```python
from build123d import *

# Parameters (mm, degrees)
CORTE_EXTRUS_O1_REACH = 512
ESBO_O2_R             = 4.5


with BuildPart() as part:
    # Esboço1 → Revolução1 (revolve)
    with BuildSketch(Plane.XY):
        Polygon((0, 510), (173, 510), (173, 500), (136.525, 500), (136.525, 0), (125.955, 0), (125.955, 10), (131.955, 10), (131.955, 500), (0, 500), align=None)
    revolve(axis=Axis((0, 0, 0), (0, 1, 0)))

    # Esboço2 → Corte-extrusão1 (cut, up to next)
    with BuildSketch(Plane(origin=(0, 510, 0), x_dir=(1, 0, 0), z_dir=(0, 1, 0)), mode=Mode.PRIVATE) as corte_extrus_o1_sk1:
        with Locations((0, 30)):
            Circle(ESBO_O2_R)
    corte_extrus_o1_tool1 = extrude(corte_extrus_o1_sk1.sketch, amount=-CORTE_EXTRUS_O1_REACH, mode=Mode.PRIVATE) & part.part
    add(corte_extrus_o1_tool1.solids().sort_by_distance((0, 510, -30))[0], mode=Mode.SUBTRACT)
    # Esboço2 → Corte-extrusão1 (cut, up to next)
    with BuildSketch(Plane(origin=(0, 510, 0), x_dir=(1, 0, 0), z_dir=(0, 1, 0)), mode=Mode.PRIVATE) as corte_extrus_o1_sk2:
        with Locations((30, 0)):
            Circle(ESBO_O2_R)
    corte_extrus_o1_tool2 = extrude(corte_extrus_o1_sk2.sketch, amount=-CORTE_EXTRUS_O1_REACH, mode=Mode.PRIVATE) & part.part
    add(corte_extrus_o1_tool2.solids().sort_by_distance((30, 510, 0))[0], mode=Mode.SUBTRACT)
    # Esboço2 → Corte-extrusão1 (cut, up to next)
    with BuildSketch(Plane(origin=(0, 510, 0), x_dir=(1, 0, 0), z_dir=(0, 1, 0)), mode=Mode.PRIVATE) as corte_extrus_o1_sk3:
        with Locations((0, -30)):
            Circle(ESBO_O2_R)
    corte_extrus_o1_tool3 = extrude(corte_extrus_o1_sk3.sketch, amount=-CORTE_EXTRUS_O1_REACH, mode=Mode.PRIVATE) & part.part
    add(corte_extrus_o1_tool3.solids().sort_by_distance((0, 510, 30))[0], mode=Mode.SUBTRACT)
    # Esboço2 → Corte-extrusão1 (cut, up to next)
    with BuildSketch(Plane(origin=(0, 510, 0), x_dir=(1, 0, 0), z_dir=(0, 1, 0)), mode=Mode.PRIVATE) as corte_extrus_o1_sk4:
        with Locations((-30, 0)):
            Circle(ESBO_O2_R)
    corte_extrus_o1_tool4 = extrude(corte_extrus_o1_sk4.sketch, amount=-CORTE_EXTRUS_O1_REACH, mode=Mode.PRIVATE) & part.part
    add(corte_extrus_o1_tool4.solids().sort_by_distance((-30, 510, 0))[0], mode=Mode.SUBTRACT)


solid = part.part
```
Geometry check sheet. Reference: the model listing, model coordinates, mm. A direction names the side the tool comes from. Coordinates: 2 decimals unless noted, no trailing zeros. Order: outer loops, then holes, each group sorted by start corner. A loop starts at its lowest first (then second) coordinate and runs counter-clockwise, first axis right, second up.
Item 1: Scan lines: line 1 along Z through (x, y) = (0, 505); line 2 along X through (y, z) = (6.5, 0) (3 decimals). Record each from-to range of solid material in increasing order.
Item 2: Section check D-D (x = 152). Enter the section's corners in (y, z), plus the area to 3 significant figures.
Item 3: Mould release check, pull along X, two halves, no side actions. Record for faces 1 (the cylindrical face through (125.86, 258.43, -39.64)), 2 (the flat face through (127, 500, -52)), 3 (the cylindrical face through (-137.287, 504.93, 105.268)): released by +X, released by -X, zero draft, split by the parting line, or undercut.
Item 4: Tool access check on faces 4 (the cylindrical face through (-136.393, 246.5, -6.003)), 5 (the flat face through (2, 510, -2)), 6 (the flat face through (-117, 10, 48)). Record the directions out of +Z, -Z, +X, -X, +Y, -Y that give a thin tool (end or side, any length) a straight path to the whole face; none if there is none.
Item 5: Section check B-B (x = -78). Enter the section's corners in (y, z).
Item 6: Section check C-C (z = 77). Enter the section's corners in (x, y), plus the area to 3 significant figures.
Item 7: Depth check by flat-ended pin: pin 1 (12 mm diameter, centred on x = 110, y = 225.5, fed in from +Z); pin 2 (8 mm diameter, centred on y = 257, z = 112.5, fed in from -X); pin 3 (3 mm diameter, centred on x = 98, y = 149, fed in from -Z); pin 4 (7 mm diameter, centred on x = 30, z = 0, fed in from +Y). Enter the tip coordinate at first touch or a pass-through.
Item 8: Section check A-A (y = 362.5). Enter the section's corners in (x, z) (3 decimals).
Check sheet entries:
1. line 1: z = -173 to -34.5, -25.5 to 25.5, 34.5 to 173
1. line 2: x = -136.525 to -125.955, 125.955 to 136.525
2. outline: (500, -82.61) - (510, -82.61) - (510, 82.61) - (500, 82.61) - close
2. area: 1,650 mm2
3. face 1: undercut
3. face 2: zero draft
3. face 3: split by the parting line
4. face 4: -Y
4. face 5: +Z, -Z, +X, -X, +Y
4. face 6: none
5. outline: (0, -112.05) - (500, -112.05) - (500, -154.42) - (510, -154.42) - (510, 154.42) - (500, 154.42) - (500, 112.05) - (0, 112.05) - (0, 98.9) - (10, 98.9) - (10, 106.43) - (500, 106.43) - (500, -106.43) - (10, -106.43) - (10, -98.9) - (0, -98.9) - close
6. outline: (-154.92, 500) - (-112.74, 500) - (-112.74, 0) - (-99.68, 0) - (-99.68, 10) - (-107.16, 10) - (-107.16, 500) - (107.16, 500) - (107.16, 10) - (99.68, 10) - (99.68, 0) - (112.74, 0) - (112.74, 500) - (154.92, 500) - (154.92, 510) - (-154.92, 510) - close
6. area: 8,830 mm2
7. pin 1: stops at z = 88.45
7. pin 2: stops at x = -82.87
7. pin 3: stops at z = -96.58
7. pin 4: passes through
8. outline: circle Ø273.05 at (0, 0); hole circle Ø263.91 at (0, 0)
